Verification items for the finished model (mm, model axes). Face numbers are marked on the shaded views. Coordinates: 2 decimals unless noted, no trailing zeros. Order: outer loops, then holes, each group sorted by start corner. A loop starts at its lowest first (then second) coordinate and runs counter-clockwise, first axis right, second up. Notation, with made-up numbers: (-33, 35.25) -> (3, 35.25) arc R6 ccw to (3, 41.25) -> close; hole circle Ø4 at (19.5, 52.25). An arc over 180 degrees is marked (long way). Write item = value, one per line. Start each with the question number.
1. Cross-section at A-A on y = 168. Record the cut outline in (x, z).
2. Release check for a two-part mould opening along Y. For the marked faces 1, 2 and 3 record: +Y half, -Y half, draft (parallel to the pull), parting line (faces both ways), or undercut.
3. Cross-section at B-B on x = -81. Record the cut outline in (y, z).
4. Cross-section at C-C on z = 15.5. Record the cut outline in (x, y), plus the area to 3 significant figures.
5. Go/stop test with flat-tipped pins: P1, Ø1.6, axis at y = 140, z = -102, coming from the -X side; P2, Ø3, axis at x = 27.5, y = 105, coming from the -Z side; P3, Ø12, axis at y = 136.5, z = -25.5, coming from the +X side; P4, Ø7, axis at x = -73.43, y = 145.5, coming from the +Z side. Record where each tip stops, or that it passes through.
6. Cross-section at D-D on x = 64.5. Record the cut outline in (y, z), plus the area to 3 significant figures.
7. Thickness scan on line 1 along Y through (x, z) = (84, -79.5); line 2 along X through (y, z) = (76.5, -56); line 3 along Y through (x, z) = (40.5, 9.5). Record the ranges inside material, lowest first. Write a range as from..to.
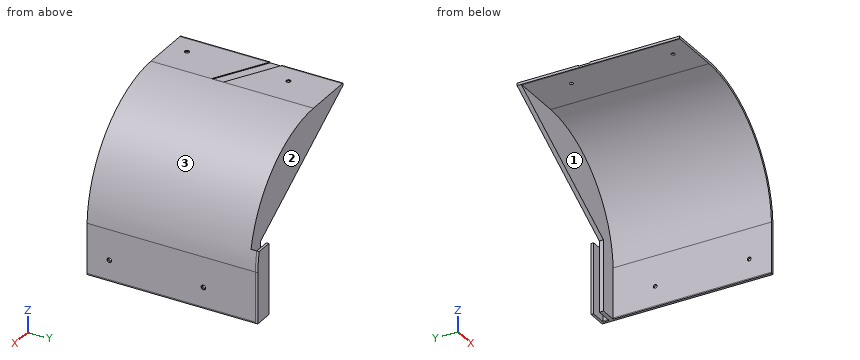
Solid Edge part; units mm, degrees
sketch "Sketch1" plane through (0, 0, 0) normal (0, -1, 0) x (1, 0, 0)
  arc A0 (-37.1299, 86.2147) -> (92.6101, -40.7853) centre (-39.0034, -45.4688) cw
  line L0 (92.6101, -40.7853) -> (92.6101, -101.2453)
  line L1 (92.6101, -101.2453) -> (95.6101, -101.2453)
  line L2 (95.6101, -101.2453) -> (95.6101, -40.7853)
  arc A1 (-37.1299, 89.2147) -> (95.6101, -40.7853) centre (-39.0019, -45.4657) cw
  line L3 (-97.1299, 89.2147) -> (-37.1299, 89.2147)
  line L4 (-97.1299, 86.2147) -> (-97.1299, 89.2147)
  line L5 (-37.1299, 86.2147) -> (-97.1299, 86.2147)
  dimension "D1" = 37.1299
  dimension "D2" = 92.6101
  dimension "D3" = 37.1299
  dimension "D4" = 95.6101
extrude "Protrusion1" add sketch "Sketch1" against normal blind 204
sketch "Sketch2" plane through (-67.1299, 85, 89.2147) normal (0, 0, 1) x (1, 0, 0)
  circle A0 centre (-6.3, -62.5) radius 2.25
  circle A1 centre (-6.3, 60.5) radius 2.25
  dimension "D1" = 6.3
extrude "Cutout1" cut sketch "Sketch2" against normal through all
sketch "Sketch3" plane through (95.6101, 85, -66.0153) normal (1, 0, 0) x (0, 1, 0)
  circle A0 centre (56, -11.65) radius 2.25
  circle A1 centre (-58, -11.65) radius 2.25
  dimension "D1" = 58
  dimension "D2" = 58
extrude "Cutout2" cut sketch "Sketch3" against normal through all
sketch "Sketch4" plane through (-97.1299, 102, 87.7147) normal (-1, 0, 0) x (0, -1, 0)
  line L0 (-102, -1.5) -> (102, -1.5)
  line L1 (102, -1.5) -> (102, 1.5)
  line L2 (102, 1.5) -> (-102, 1.5)
  line L3 (-102, 1.5) -> (-102, -1.5)
extrude "Extrusionsausprägung_3" add sketch "Sketch4" along normal blind 1.3
sketch "Sketch5" plane through (94.1101, 102, -101.2453) normal (0, 0, -1) x (0, 1, 0)
  line L0 (-102, 1.5) -> (102, 1.5)
  line L1 (102, 1.5) -> (102, -1.5)
  line L2 (102, -1.5) -> (-102, -1.5)
  line L3 (-102, -1.5) -> (-102, 1.5)
extrude "Extrusionsausprägung_4" add sketch "Sketch5" along normal blind 1.42
sketch "Sketch6" plane through (-67.7799, 102, 89.2147) normal (0, 0, 1) x (0, 1, 0)
  line L0 (21.17, 30.65) -> (-14.2216, -30.65)
  line L1 (-14.2216, -30.65) -> (-28.6553, -30.65)
  line L2 (-28.6553, -30.65) -> (6.7362, 30.65)
  line L3 (6.7362, 30.65) -> (21.17, 30.65)
  dimension "D1" = 21.17
extrude "Cutout3" cut sketch "Sketch6" against normal blind 1
chamfer "Fase_1" distance 0.5 angle 60 4 edges at (-75.6799, 22.5, 89.2147) (-75.6799, 145.5, 89.2147) (95.6101, 24.75, -77.6653) (95.6101, 138.75, -77.6653) measured on face at (-87.7299, 88.9082, 89.2147) measured on face at (-87.7299, 183.4675, 89.2147) measured on face at (-87.7299, 88.9082, 89.2147) measured on face at (-87.7299, 183.4675, 89.2147) measured on face at (95.6101, 167.96, -91.7732)
sketch "Sketch7" plane through (-67.7799, 145.8892, 89.2147) normal (0, 0, 1) x (-1, 0, 0)
  line L0 (30.65, -58.1108) -> (-160.39, -58.1108)
  line L1 (-160.39, -58.1108) -> (-160.39, -53.1108)
  line L2 (-160.39, -53.1108) -> (30.65, -53.1108)
  line L3 (30.65, -53.1108) -> (30.65, -58.1108)
  dimension "D1" = 30.65
  dimension "D2" = 30.65
extrude "Cutout4" cut sketch "Sketch7" against normal up to next
sketch "Sketch8" plane through (94.1101, 204, -59.7426) normal (0, 1, 0) x (0, 0, -1)
  line L0 (-42.9227, 1.5) -> (42.9227, 1.5)
  line L1 (42.9227, 1.5) -> (42.9227, -1.5)
  line L2 (42.9227, -1.5) -> (-18.9573, -1.5)
  arc A0 (-18.9573, -1.5) -> (-42.9227, 1.5) centre (-14.2769, 133.1121) cw
extrude "Extrusionsausprägung_7" add sketch "Sketch8" along normal blind 3
sketch "Sketch9" plane through (92.6101, 103.5, -59.7426) normal (-1, 0, 0) x (0, -1, 0)
  line L0 (-88.5, 42.9227) -> (-93.5, 42.9227)
  line L1 (-93.5, 42.9227) -> (-93.5, -42.9227)
  line L2 (-93.5, -42.9227) -> (-88.5, -42.9227)
  line L3 (-88.5, -42.9227) -> (-88.5, 42.9227)
  line L4 (-103.5, 42.9227) -> (-100.5, 42.9227)
  line L5 (-100.5, 42.9227) -> (-100.5, -42.9227)
  line L6 (-100.5, -42.9227) -> (-103.5, -42.9227)
  line L7 (-103.5, -42.9227) -> (-103.5, 42.9227)
  dimension "D1" = 100.5
  dimension "D2" = 93.5
  dimension "D3" = 88.5
extrude "Extrusionsausprägung_8" add sketch "Sketch9" along normal blind 20
sketch "Sketch10" plane through (84.1101, 103.5, -102.6653) normal (0, 0, -1) x (0, 1, 0)
  line L0 (93.5, 8.5) -> (93.5, -182.54)
  line L1 (93.5, -182.54) -> (97, -182.54)
  line L2 (97, -182.54) -> (97, 8.5)
  line L3 (97, 8.5) -> (93.5, 8.5)
extrude "Cutout5" cut sketch "Sketch10" against normal up to next
sketch "Sketch11" plane through (-2.9099, 197, -6.7253) normal (0, 1, 0) x (-1, 0, 0)
  line L0 (95.52, 92.94) -> (-75.52, -10.0947)
  line L1 (-92.4495, -10.0947) -> (-75.52, -10.0947)
  arc A0 (34.22, 92.94) -> (-92.4495, -10.0947) centre (36.0936, -38.7436) ccw
  line L2 (95.52, 92.94) -> (34.22, 92.94)
extrude "Protrusion2" add sketch "Sketch11" against normal up to vertex (5 mm away)
properties material "Nylon, allgemein"
Worked out:
q1.outline = (-98.43, 86.21) -> (-97.13, 86.21) -> (-37.13, 86.21) arc R131.7 cw to (92.61, -40.79) -> (92.61, -101.25) -> (92.61, -102.67) -> (95.61, -102.67) -> (95.61, -101.25) -> (95.61, -40.79) arc R134.69 ccw to (-37.13, 89.21) -> (-97.13, 89.21) -> (-98.43, 89.21) -> close
q2.face_1 = -Y half
q2.face_2 = undercut
q2.face_3 = draft
q3.outline = (0, 86.21) -> (192, 86.21) -> (192, 75.71) -> (197, 75.71) -> (197, 89.21) -> (113.11, 89.21) -> (113.11, 88.21) -> (98.67, 88.21) -> (98.67, 89.21) -> (0, 89.21) -> close
q4.outline = (18.96, 192) -> (77.73, 192) -> (77.73, 0) -> (81.1, 0) -> (81.1, 197) -> (18.96, 197) -> close
q4.area = 958 mm²
q5.P1 = 92.61
q5.P2 = 67.31
q5.P3 = 94.97
q5.P4 = 89.21
q6.outline = (0, 35.96) -> (192, 35.96) -> (192, -11.93) -> (197, -11.93) -> (197, 40.73) -> (0, 40.73) -> close
q6.area = 1,180 mm²
q7.line_1 = 192..197, 204..207
q7.line_2 = 92.61..95.61
q7.line_3 = 192..197
